Verification items for the finished model (mm, model axes). Face numbers are marked on the shaded views. A direction names the side the tool comes from. Round coordinates to 2 decimals unless told otherwise and drop trailing zeros. Order: outer loops, then holes, each group sorted by start corner. A loop starts at its lowest first (then second) coordinate and runs counter-clockwise, first axis right, second up. Notation, with made-up numbers: (68.5, -5.5) -> (115.5, -5.5) arc R13 ccw to (115.5, 6.5) -> close; hole circle Ø11 at (61.25, 87). An arc over 180 degrees is marked (long way). Put each result on its own line as item: value.
```python
from build123d import *

# Parameters (mm, degrees)
SKETCH_1_W                  = 320
SKETCH_1_H                  = 200
SM_BASE_FLANGE_1_DEPTH      = 4
HOLE_WIZARD_1_AT_2_COUNT    = 2
HOLE_WIZARD_1_AT_2_PITCH    = 30
HOLE_WIZARD_1_AT_3_COUNT    = 2
HOLE_WIZARD_1_AT_3_PITCH    = 43.863424399
HOLE_WIZARD_1_AT_4_COUNT    = 2
HOLE_WIZARD_1_AT_4_PITCH    = 32
HOLE_WIZARD_1_AT_5_COUNT    = 2
HOLE_WIZARD_1_AT_5_PITCH    = 129.031004026
HOLE_WIZARD_1_AT_6_COUNT    = 2
HOLE_WIZARD_1_AT_6_PITCH    = 125
HOLE_WIZARD_1_AT_7_COUNT    = 2
HOLE_WIZARD_1_AT_7_PITCH    = 158.268758762
HOLE_WIZARD_1_AT_8_COUNT    = 2
HOLE_WIZARD_1_AT_8_PITCH    = 155
SKETCH_9_W                  = 30
SKETCH_9_H                  = 45
SM_BASE_FLANGE_1_2_DEPTH    = 4
SKETCH_27_W                 = 89
SKETCH_27_H                 = 5
CUT_EXTRUDE_2_DEPTH         = 216.965274987
SM_EDGE_FLANGE_1_DEPTH      = 100
SM_EDGE_FLANGE_1_BEND_DEPTH = 100
HOLE_START                  = -108.5
HOLE_WIZARD_8_2_8_2_1_DEPTH = 217
F_5_2_5_2_DIAMETER_HOLE1_D  = 5.2
CUT_EXTRUDE_1_REACH         = 223.199
SKETCH_21_W                 = 30
SKETCH_21_H                 = 30
HOLE_WIZARD_M3_2_D          = 2.5
OTHER_START                 = -108.5
OTHER_1_DEPTH               = 217
OTHER_START_2               = -4
OTHER_2_DEPTH               = 4
OTHER_2_2_DEPTH             = 4
HOLE_WIZARD_M3_1_D          = 2.5
HOLE_WIZARD_M3_3_D          = 2.5


# Read off the part's stored shape, not the designer's step: Ø8.2 (8.2) 直径槽口1, 断开-边角1, 断开-边角2
# Sheet-metal steps are written as plain solids
with BuildPart() as part:
    # Sketch 1 → Sm Base Flange 1 (new body)
    with BuildSketch(Plane(origin=(0, 0, 0), x_dir=(1, 0, 0), z_dir=(0, 1, 0))):
        Rectangle(SKETCH_1_W, SKETCH_1_H)
    extrude(amount=-SM_BASE_FLANGE_1_DEPTH)

    # 草图7 → 打孔尺寸开槽半沉头螺钉的类型1 (revolve, cut)
    with BuildSketch(Plane(origin=(-154, 0, 62.5), x_dir=(0, 0, 1), z_dir=(1, 0, 0))):
        Polygon((0, 0), (0, 4), (2.75, 4), (2.75, 2.55), (5.3, 0), align=None)
    hole_wizard_1 = revolve(axis=Axis((-154, 6.35, 62.5), (0, -1, 0)), mode=Mode.SUBTRACT)

    # 打孔尺寸开槽半沉头螺钉的类型1 at 2: 打孔尺寸开槽半沉头螺钉的类型1 ×2
    with Locations(*[(0, 0, i * HOLE_WIZARD_1_AT_2_PITCH) for i in range(1, HOLE_WIZARD_1_AT_2_COUNT)]):
        add(hole_wizard_1, mode=Mode.SUBTRACT)

    # 打孔尺寸开槽半沉头螺钉的类型1 at 3: 打孔尺寸开槽半沉头螺钉的类型1 ×2
    with Locations(*[Vector(0.7295372041400852, 0, 0.6839411288813297) * (i * HOLE_WIZARD_1_AT_3_PITCH) for i in range(1, HOLE_WIZARD_1_AT_3_COUNT)]):
        add(hole_wizard_1, mode=Mode.SUBTRACT)

    # 打孔尺寸开槽半沉头螺钉的类型1 at 4: 打孔尺寸开槽半沉头螺钉的类型1 ×2
    with Locations(*[(i * HOLE_WIZARD_1_AT_4_PITCH, 0, 0) for i in range(1, HOLE_WIZARD_1_AT_4_COUNT)]):
        add(hole_wizard_1, mode=Mode.SUBTRACT)

    # 打孔尺寸开槽半沉头螺钉的类型1 at 5: 打孔尺寸开槽半沉头螺钉的类型1 ×2
    with Locations(*[Vector(0.24800241028513723, 0, -0.9687594151763185) * (i * HOLE_WIZARD_1_AT_5_PITCH) for i in range(1, HOLE_WIZARD_1_AT_5_COUNT)]):
        add(hole_wizard_1, mode=Mode.SUBTRACT)

    # 打孔尺寸开槽半沉头螺钉的类型1 at 6: 打孔尺寸开槽半沉头螺钉的类型1 ×2
    with Locations(*[(0, 0, -i * HOLE_WIZARD_1_AT_6_PITCH) for i in range(1, HOLE_WIZARD_1_AT_6_COUNT)]):
        add(hole_wizard_1, mode=Mode.SUBTRACT)

    # 打孔尺寸开槽半沉头螺钉的类型1 at 7: 打孔尺寸开槽半沉头螺钉的类型1 ×2
    with Locations(*[Vector(0.20218772327747656, 0, -0.979346784625278) * (i * HOLE_WIZARD_1_AT_7_PITCH) for i in range(1, HOLE_WIZARD_1_AT_7_COUNT)]):
        add(hole_wizard_1, mode=Mode.SUBTRACT)

    # 打孔尺寸开槽半沉头螺钉的类型1 at 8: 打孔尺寸开槽半沉头螺钉的类型1 ×2
    with Locations(*[(0, 0, -i * HOLE_WIZARD_1_AT_8_PITCH) for i in range(1, HOLE_WIZARD_1_AT_8_COUNT)]):
        add(hole_wizard_1, mode=Mode.SUBTRACT)

    # 草图9 → Sm Base Flange 1 2 (add)
    with BuildSketch(Plane(origin=(0, 0, 0), x_dir=(1, 0, 0), z_dir=(0, 1, 0))):
        with Locations((-44, 122.5)):
            Rectangle(SKETCH_9_W, SKETCH_9_H)
    extrude(amount=-SM_BASE_FLANGE_1_2_DEPTH)

    # 草图27 → 切除-拉伸2 (cut, through all)
    with BuildSketch(Plane(origin=(0, 0, 0), x_dir=(1, 0, 0), z_dir=(0, 1, 0))):
        with Locations((15.5, 97.5)):
            Rectangle(SKETCH_27_W, SKETCH_27_H)
        with Locations((15.5, -97.5)):
            Rectangle(SKETCH_27_W, SKETCH_27_H)
    extrude(amount=-CUT_EXTRUDE_2_DEPTH, mode=Mode.SUBTRACT)

    # 边线-法兰1 section (across the edge) → 边线-法兰1 (add)
    with BuildSketch(Plane(origin=(60, 0, 104.5), x_dir=(0, 0, -1), z_dir=(1, 0, 0))):
        with BuildLine():
            Line((-4, 0.5), (-4, 48))
            Line((-4, 48), (0, 48))
            Line((0, 48), (0, 0.5))
            ThreePointArc((0, 0.5), (0.146446609, 0.146446609), (0.5, 0))
            Line((0.5, 0), (4.5, 0))
            Line((4.5, 0), (4.5, -4))
            Line((4.5, -4), (0.5, -4))
            ThreePointArc((0.5, -4), (-2.681980515, -2.681980515), (-4, 0.5))
        make_face()
    extrude(amount=SM_EDGE_FLANGE_1_DEPTH)

    # 边线-法兰1 section 2 (across the edge) → 边线-法兰1 bend (add)
    with BuildSketch(Plane(origin=(160, 0, -104.5), x_dir=(0, 0, 1), z_dir=(-1, 0, 0))):
        with BuildLine():
            Line((-4, 0.5), (-4, 48))
            Line((-4, 48), (0, 48))
            Line((0, 48), (0, 0.5))
            ThreePointArc((0, 0.5), (0.146446609, 0.146446609), (0.5, 0))
            Line((0.5, 0), (4.5, 0))
            Line((4.5, 0), (4.5, -4))
            Line((4.5, -4), (0.5, -4))
            ThreePointArc((0.5, -4), (-2.681980515, -2.681980515), (-4, 0.5))
        make_face()
    extrude(amount=SM_EDGE_FLANGE_1_BEND_DEPTH)

    # Ø8.2 (8.2) 直径槽口1 outline → Ø8.2 (8.2) 直径槽口1 (cut)
    with BuildSketch(Plane.XY.offset(HOLE_START)):
        with BuildLine():
            ThreePointArc((145.9, 24.6), (150, 20.5), (154.1, 24.6))
            Line((154.1, 24.6), (154.1, 36.4))
            ThreePointArc((154.1, 36.4), (150, 40.5), (145.9, 36.4))
            Line((145.9, 36.4), (145.9, 24.6))
        make_face()
        with BuildLine():
            ThreePointArc((65.9, 24.6), (70, 20.5), (74.1, 24.6))
            Line((74.1, 24.6), (74.1, 36.4))
            ThreePointArc((74.1, 36.4), (70, 40.5), (65.9, 36.4))
            Line((65.9, 36.4), (65.9, 24.6))
        make_face()
    extrude(amount=HOLE_WIZARD_8_2_8_2_1_DEPTH, mode=Mode.SUBTRACT)

    # Ø5.2 (5.2) Diameter Hole1 (through all)
    with Locations(Plane(origin=(0, 0, 0), x_dir=(1, 0, 0), z_dir=(0, 1, 0))):
        with Locations((-44, 117.5), (-44, 137.5)):
            Hole(F_5_2_5_2_DIAMETER_HOLE1_D / 2)

    # 草图21 → 切除-拉伸1 (cut, up to next)
    with BuildSketch(Plane(origin=(0, 0, 0), x_dir=(1, 0, 0), z_dir=(0, 1, 0)), mode=Mode.PRIVATE) as cut_extrude_1_sk1:
        with Locations((-85, 0)):
            Rectangle(SKETCH_21_W, SKETCH_21_H)
    cut_extrude_1_tool1 = extrude(cut_extrude_1_sk1.sketch, amount=-CUT_EXTRUDE_1_REACH, mode=Mode.PRIVATE) & part.part
    add(cut_extrude_1_tool1.solids().sort_by_distance((-85, 0, 0))[0], mode=Mode.SUBTRACT)

    # M3 螺纹孔2 (through all)
    with Locations(Plane(origin=(0, 0, 0), x_dir=(1, 0, 0), z_dir=(0, 1, 0))):
        with Locations((-106, 6), (-106, -6)):
            Hole(HOLE_WIZARD_M3_2_D / 2)

    # Other 1 outline → Other 1 (cut)
    with BuildSketch(Plane.XY.offset(OTHER_START)):
        with BuildLine():
            ThreePointArc((60, 43), (61.464466094, 46.535533906), (65, 48))
            Line((65, 48), (60, 48))
            Line((60, 48), (60, 43))
        make_face()
        with BuildLine():
            ThreePointArc((155, 48), (158.535533906, 46.535533906), (160, 43))
            Line((160, 43), (160, 48))
            Line((160, 48), (155, 48))
        make_face()
    extrude(amount=OTHER_1_DEPTH, mode=Mode.SUBTRACT)

    # Other 2 outline → Other 2 (cut)
    with BuildSketch(Plane(origin=(0, 0, 0), x_dir=(1, 0, 0), z_dir=(0, 1, 0)).offset(OTHER_START_2)):
        with BuildLine():
            Line((-29, 145), (-34, 145))
            ThreePointArc((-34, 145), (-30.464466094, 143.535533906), (-29, 140))
            Line((-29, 140), (-29, 145))
        make_face()
        with BuildLine():
            Line((-59, 145), (-59, 140))
            ThreePointArc((-59, 140), (-57.535533906, 143.535533906), (-54, 145))
            Line((-54, 145), (-59, 145))
        make_face()
        with BuildLine():
            Line((-160, 100), (-160, 95))
            ThreePointArc((-160, 95), (-158.535533906, 98.535533906), (-155, 100))
            Line((-155, 100), (-160, 100))
        make_face()
        with BuildLine():
            Line((-160, -100), (-155, -100))
            ThreePointArc((-155, -100), (-158.535533906, -98.535533906), (-160, -95))
            Line((-160, -95), (-160, -100))
        make_face()
    extrude(amount=OTHER_2_DEPTH, mode=Mode.SUBTRACT)

    # Other 2 2 outline → Other 2 2 (add)
    with BuildSketch(Plane(origin=(0, 0, 0), x_dir=(1, 0, 0), z_dir=(0, 1, 0)).offset(OTHER_START_2)):
        with BuildLine():
            Line((-29, -95), (-29, -100))
            ThreePointArc((-29, -100), (-27.535533906, -96.464466094), (-24, -95))
            Line((-24, -95), (-29, -95))
        make_face()
        with BuildLine():
            ThreePointArc((-24, 95), (-27.535533906, 96.464466094), (-29, 100))
            Line((-29, 100), (-29, 95))
            Line((-29, 95), (-24, 95))
        make_face()
        with BuildLine():
            ThreePointArc((-59, 105), (-60.464466094, 101.464466094), (-64, 100))
            Line((-64, 100), (-59, 100))
            Line((-59, 100), (-59, 105))
        make_face()
    extrude(amount=OTHER_2_2_DEPTH)

    # M3 螺纹孔1 (through all)
    with Locations(Plane(origin=(0, 0, 0), x_dir=(1, 0, 0), z_dir=(0, 1, 0))):
        with Locations((11, 88), (-6, 88)):
            Hole(HOLE_WIZARD_M3_1_D / 2)

    # M3 螺纹孔3 (through all)
    with Locations(Plane(origin=(0, 0, 0), x_dir=(1, 0, 0), z_dir=(0, 1, 0))):
        with Locations((-54, 133.5), (-54, 121.5)):
            Hole(HOLE_WIZARD_M3_3_D / 2)


solid = part.part
```
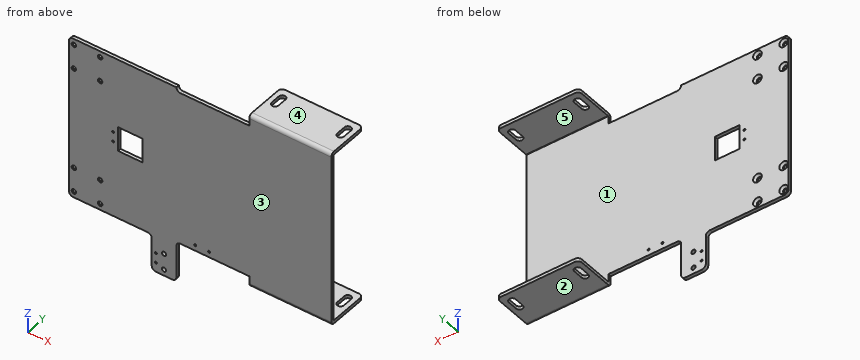
Item 1: Sectioned sample at D-D, the plane x = 54.5. Record the boundary of the cut face in (y, z), then the cut area to 3 significant figures.
Geometry check:
outline: (-4, -95) -> (0, -95) -> (0, 95) -> (-4, 95) -> close
area: 760 mm2
Item 2: Sectioned sample at A-A, the plane y = 16.5. Record the boundary of the cut face in (x, z), then the cut area to 3 significant figures.
Geometry check:
outline: (60, -108.5) -> (160, -108.5) -> (160, -104.5) -> (60, -104.5) -> close; (60, 104.5) -> (160, 104.5) -> (160, 108.5) -> (60, 108.5) -> close
area: 800 mm2
Item 3: Release check for a two-part mould opening along Z. For the marked faces 1, 2 and 3 record: pulls with the +Z half, pulls with the -Z half, needs draft (parallel to the pull), parting line crosses it, or undercut.
Geometry check:
face 1: undercut
face 2: pulls with the -Z half
face 3: needs draft
Item 4: Sectioned sample at B-B, the plane x = 150. Record the boundary of the cut face in (y, z), then the cut area to 3 significant figures.
Geometry check:
outline: (-4, -104) arc R4.5 ccw to (0.5, -108.5) -> (20.5, -108.5) -> (20.5, -104.5) -> (0.5, -104.5) arc R0.5 cw to (0, -104) -> (0, 104) arc R0.5 cw to (0.5, 104.5) -> (20.5, 104.5) -> (20.5, 108.5) -> (0.5, 108.5) arc R4.5 ccw to (-4, 104) -> close; (40.5, -108.5) -> (48, -108.5) -> (48, -104.5) -> (40.5, -104.5) -> close; (40.5, 104.5) -> (48, 104.5) -> (48, 108.5) -> (40.5, 108.5) -> close
area: 1,080 mm2
Item 5: Depth check by flat-ended pin: pin 1 Ø5 at (x, z) = (-122, 92.5) entering from -Y; pin 2 Ø12 at (x, z) = (95.5, 72.5) entering from +Y; pin 3 Ø2 at (y, z) = (32.5, -106) entering from -X; pin 4 Ø3 at (x, y) = (13, -1.5) entering from +Z. Enter the tip coordinate at first touch or a pass-through.
Geometry check:
pin 1: through
pin 2: y = 0
pin 3: x = 60
pin 4: z = 95
Item 6: Sectioned sample at C-C, the plane z = 36. Record the boundary of the cut face in (x, y), then the cut area to 3 significant figures.
Geometry check:
outline: (-160, -4) -> (160, -4) -> (160, 0) -> (-160, 0) -> close
area: 1,280 mm2
Item 7: Material ranges on line 1 along X through (y, z) = (-3.6, -62.5); line 2 along Z through (x, y) = (88, 6); line 3 along Y through (x, z) = (35, 48.5), recorded low to high.
Geometry check:
line 1: -160 to -156.75, -151.25 to -124.75, -119.25 to 160
line 2: -108.5 to -104.5, 104.5 to 108.5
line 3: -4 to 0
Item 8: Tool access check on the marked faces 4 and 5. Record the directions out of +Z, -Z, +X, -X, +Y, -Y that give a thin tool (end or side, any length) a straight path to the whole face; none if there is none.
Geometry check:
face 4: +Z, +X, -X, +Y, -Y
face 5: +X, -X, +Y
